```python
from build123d import *

# Parameters (mm, degrees)
SKETCH2_R          = 5
CUT_EXTRUDE1_DEPTH = 54.768020235
SKETCH3_W          = 3
SKETCH3_H          = 2
CUT_EXTRUDE2_DEPTH = 54.768020235


with BuildPart() as part:
    # Sketch1 → Revolve2 (revolve)
    with BuildSketch(Plane.XY, mode=Mode.PRIVATE) as revolve2_sk:
        Polygon((34, 14.5), (34, 1.5), (24, 1.5), (24, 0), (0, 0), (0, 21), (15, 21), (15, 16), (35, 16), (35, 14.5), align=None)
    revolve(revolve2_sk.sketch.rotate(Axis((0, 0, 0), (0, 1, 0)), 90), axis=Axis((0, 0, 0), (0, 1, 0)))

    # Sketch2 → Cut-Extrude1 (cut, through all)
    with BuildSketch(Plane(origin=(0, 21, 0), x_dir=(1, 0, 0), z_dir=(0, 1, 0))):
        with Locations(Location((0, 0, 0), (0, 0, 270))):
            Circle(SKETCH2_R)
    extrude(amount=-CUT_EXTRUDE1_DEPTH, mode=Mode.SUBTRACT)

    # Sketch3 → Cut-Extrude2 (cut, through all)
    with BuildSketch(Plane(origin=(0, 21, 0), x_dir=(1, 0, 0), z_dir=(0, 1, 0))):
        with Locations((0, -5.3)):
            Rectangle(SKETCH3_W, SKETCH3_H)
    extrude(amount=-CUT_EXTRUDE2_DEPTH, mode=Mode.SUBTRACT)


solid = part.part
```
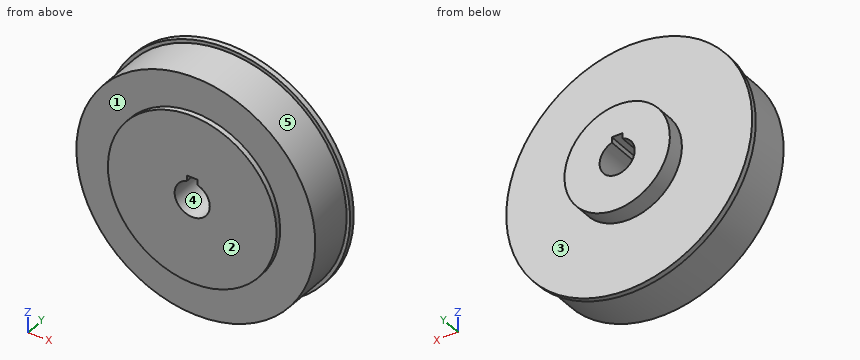
Work out the finished part from the listing and answer in its coordinate system (mm). Face numbers are marked on the shaded views. A direction names the side the tool comes from. Round coordinates to 2 decimals unless told otherwise and drop trailing zeros. Loops run counter-clockwise (first coordinate to the right, second up) from the corner with the lowest first, then second, coordinate; pieces in that order, holes last. Notation, with made-up numbers: (6, 36.25) -> (39, 36.25) arc R19 cw to (39, 52.25) -> close; hole circle Ø1 at (80.5, -12). An arc over 180 degrees is marked (long way). Write each question's results on one line, items separated by ' | '. Start each with the question number.
1. Section B-B (x = 0) is taken. Determine the outline of the cut face in (y, z).
2. Section A-A (z = 0) is taken. Determine the outline of the cut face in (x, y).
3. Section D-D (z = -18) is taken. Determine the outline of the cut face in (x, y), plus the area to 3 significant figures.
4. Given pin 1 Ø10 at (x, z) = (-16, -13.5) entering from -Y; pin 2 Ø4 at (y, z) = (7.5, -21.5) entering from -X; pin 3 Ø4 at (x, y) = (-11, 9) entering from +Z; pin 4 Ø10 at (x, y) = (-20, 7) entering from -Z, each flat-ended and moving along its own axis, determine where each tip first touches the part or whether it passes through.
5. Section C-C (y = 18.5) is taken. Determine the outline of the cut face in (x, z), plus the area to 3 significant figures.
6. Find the intervals of material crossed by probe 1 along X at (y, z) = (8, 0); probe 2 along Y at (x, z) = (-22.5, -19.5); probe 3 along Y at (x, z) = (-13, 11), in increasing order. Write a range as from..to.
7. For a pull along Z with two mould halves and no side action, classify the marked faces 3, 4 and 5 as +Z half, -Z half, draft (parallel to the pull), parting line (faces both ways), or undercut.
8. A tool of negligible diameter and unlimited length cuts with its end or side. For the marked faces 1 and 2, from which of +Z, -Z, +X, -X, +Y, -Y can it reach the whole face along a straight path? Write none if from no direction.
Evaluation:
1) outline: (0, -24) -> (1.5, -24) -> (1.5, -34) -> (14.5, -34) -> (14.5, -35) -> (16, -35) -> (16, -15) -> (21, -15) -> (21, -5) -> (0, -5) -> close; (0, 6.3) -> (21, 6.3) -> (21, 15) -> (16, 15) -> (16, 35) -> (14.5, 35) -> (14.5, 34) -> (1.5, 34) -> (1.5, 24) -> (0, 24) -> close
2) outline: (-35, 14.5) -> (-34, 14.5) -> (-34, 1.5) -> (-24, 1.5) -> (-24, 0) -> (-5, 0) -> (-5, 21) -> (-15, 21) -> (-15, 16) -> (-35, 16) -> close; (5, 0) -> (24, 0) -> (24, 1.5) -> (34, 1.5) -> (34, 14.5) -> (35, 14.5) -> (35, 16) -> (15, 16) -> (15, 21) -> (5, 21) -> close
3) outline: (-30.02, 14.5) -> (-28.84, 14.5) -> (-28.84, 1.5) -> (-15.87, 1.5) -> (-15.87, 0) -> (15.87, 0) -> (15.87, 1.5) -> (28.84, 1.5) -> (28.84, 14.5) -> (30.02, 14.5) -> (30.02, 16) -> (-30.02, 16) -> close | area: 888 mm2
4) pin 1: stops at y = 0 | pin 2: stops at x = -27.85 | pin 3: stops at z = 32.79 | pin 4: stops at z = -30.51
5) outline: circle Ø30 at (0, 0); hole (-1.5, 4.77) arc R5 ccw (long way) to (1.5, 4.77) -> (1.5, 6.3) -> (-1.5, 6.3) -> close | area: 624 mm2
6) probe 1: x = -34..-5, 5..34 | probe 2: y = 1.5..16 | probe 3: y = 0..16
7) face 3: draft | face 4: undercut | face 5: parting line
8) face 1: -Y | face 2: +Z, -Z, +X, -X, -Y
